Autodesk Inventor part; units mm, degrees
ref_plane "Work Plane1" through (10, 0, 0) normal (1, 0, 0) x (0, 0, -1)
ref_plane "YZ Plane" through (0, 0, 0) normal (1, 0, 0) x (0, 1, 0)
ref_plane "XZ Plane" through (0, 0, 0) normal (0, 1, 0) x (-1, 0, 0)
sketch "Sketch1" plane through (0, 0, 0) normal (0, 0, 1) x (1, 0, 0)
  line L0 (0, 0) -> (20, 0)
  line L1 (20, 0) -> (20, 31)
  line L2 (20, 31) -> (0, 31)
  line L3 (0, 31) -> (0, 0)
  dimension "d0" = 20
  dimension "d1" = 31
extrude "Extrusion1" add sketch "Sketch1" along normal blind 7
sketch "Sketch2" plane through (0, 0, 7) normal (0, 0, 1) x (1, 0, 0)
  line L0 (20, 31) -> (0, 31)
  line L1 (2, 31) -> (18, 31)
  line L2 (18, 31) -> (18, 11)
  line L3 (18, 11) -> (2, 11)
  line L4 (2, 11) -> (2, 31)
  line L5 (0, 31) -> (0, 0)
  line L6 (20, 0) -> (20, 31)
  dimension "d4" = 20
  dimension "d5" = 2
  dimension "d6" = 2
extrude "Extrusion2" cut sketch "Sketch2" against normal blind 4.5
sketch "Sketch3" plane through (0, 0, 7) normal (0, 0, 1) x (1, 0, 0)
  line L0 (18, 11) -> (2, 11)
  line L1 (1, 0) -> (19, 0)
  line L2 (19, 0) -> (19, 11)
  line L3 (19, 11) -> (1, 11)
  line L4 (1, 11) -> (1, 0)
  line L5 (0, 31) -> (0, 0)
  line L6 (20, 0) -> (20, 31)
  dimension "d9" = 1
  dimension "d10" = 1
extrude "Extrusion3" cut sketch "Sketch3" against normal blind 3
sketch "Sketch4" plane through (0, 0, 2.5) normal (0, 0, 1) x (1, 0, 0)
  circle A0 centre (6.19, 15) radius 1.5
  circle A1 centre (13.81, 15) radius 1.5
  line L0 (19, 0) -> (1, 0)
  line L1 (2, 31) -> (18, 31)
  line L2 (2, 11) -> (2, 31) construction
  line L3 (2, 31) -> (18, 31) construction
  line L4 (2, 11) -> (2, 31) construction
  line L5 (18, 11) -> (2, 11) construction
  line L6 (18, 31) -> (18, 11) construction
  line L7 (20, 31) -> (0, 31) construction
  line L8 (10, 31) -> (10, 11) construction
  line L9 (18, 11) -> (2, 11) construction
  line L10 (10, 31) -> (30, 31) construction
  point P0 (0, 0)
  point P1 (2, 21)
  dimension "d13" = 3
  dimension "d14" = 3
  dimension "d15" = 7.62
  dimension "d16" = 15
  dimension "d17" = 90
extrude "Extrusion4" cut sketch "Sketch4" against normal up to next
chamfer "Chamfer1" distance 0.5 angle 45 2 edges at (4.69, 15, 2.5) (12.31, 15, 2.5)
sketch "Sketch5" plane through (20, 0, 0) normal (1, 0, 0) x (0, 0, -1)
  line L0 (0, 0) -> (-7, 0) construction
  line L1 (-3.5, 0) -> (-3.5, 31) construction
  line L2 (-3.5, 0) -> (27.5, 0) construction
  line L3 (-3.5, 5) -> (-3.5, 10) construction
  line L4 (-2, 5) -> (-2, 10)
  line L5 (-5, 10) -> (-5, 5)
  arc A0 (-5, 5) -> (-2, 5) centre (-3.5, 5) ccw
  arc A1 (-2, 10) -> (-5, 10) centre (-3.5, 10) ccw
  line L6 (-3.5, 21) -> (-3.5, 26) construction
  line L7 (-2, 21) -> (-2, 26)
  line L8 (-5, 26) -> (-5, 21)
  arc A2 (-5, 21) -> (-2, 21) centre (-3.5, 21) ccw
  arc A3 (-2, 26) -> (-5, 26) centre (-3.5, 26) ccw
  line L9 (0, 31) -> (-7, 31)
  point P0 (-3.5, 7.5)
  point P1 (-3.5, 23.5)
  dimension "d23" = 31
  dimension "d24" = 90
  dimension "d25" = 3
  dimension "d26" = 3
  dimension "d27" = 5
  dimension "d28" = 5
  dimension "d29" = 5
  dimension "d30" = 5
extrude "Extrusion5" add sketch "Sketch5" along normal blind 1
ref_plane "Work Plane1" through (10, 0, 0) normal (1, 0, 0) x (0, 0, -1)
mirror "Mirror1" about plane through (10, 0, 0) normal (1, 0, 0) of "Extrusion5"
fillet "Fillet2" radius 1 16 edges at (21, 19.5, 3.5) (21, 23.5, 2) (21, 27.5, 3.5) (21, 23.5, 5) (21, 3.5, 3.5) (21, 7.5, 2) (21, 11.5, 3.5) (21, 7.5, 5) (-1, 19.5, 3.5) (-1, 23.5, 2) (-1, 27.5, 3.5) (-1, 23.5, 5) (-1, 3.5, 3.5) (-1, 7.5, 2) (-1, 11.5, 3.5) (-1, 7.5, 5)
fillet "Fillet3" radius 1 2 edges at (2, 21, 2.5) (18, 21, 2.5)
chamfer "Chamfer2" distance 0.5 angle 45 2 edges at (12.31, 15, 0) (4.69, 15, 0)
properties part number "Top"
CAD build for the part. Positions are in the model's coordinates, mm. A direction names the side the tool comes from. Give positions to 0.01 mm unless a question says otherwise; leave off trailing zeros. Loops run counter-clockwise (first coordinate to the right, second up) from the corner with the lowest first, then second, coordinate; pieces in that order, holes last. Notation, with made-up numbers: (30, -31) -> (65, -31) arc R11 cw to (65, -25) -> close; hole circle Ø7 at (34.5, 71.5). An arc over 180 degrees is marked (long way). Use a Markdown table: item, result.
1. Which spindle directions (+Z, -Z, +X, -X, +Y, -Y) get a long thin tool onto all of the face, cutting with end or side? Do faces 1 (the flat face through (18.5, 11, 5.5)), 2 (the flat face through (21, 23.5, 3.5)). Say none if no direction does.
Check result:
| item | result |
|---|---|
| face 1 | +Z, -Y |
| face 2 | +Z, -Z, +X, +Y, -Y |
2. Flat gauge pins, fed straight in: pin 1 (0.8 mm diameter, centred on x = 12, z = 3, fed in from +Y); pin 2 (0.8 mm diameter, centred on x = 1.5, z = 6, fed in from -Y); pin 3 (0.9 mm diameter, centred on y = 6, z = 6, fed in from +X); pin 4 (1.8 mm diameter, centred on x = 13.81, y = 15, fed in from +Z). Where does each tip first touch, or does it go through?
Check result:
| item | result |
|---|---|
| pin 1 | stops at y = 11 |
| pin 2 | stops at y = 11 |
| pin 3 | stops at x = 20 |
| pin 4 | passes through |
3. Slice it at B-B (y = 15). List the corners of the cut face in (x, z).
Check result:
| item | result |
|---|---|
| outline | (0, 0) -> (4.19, 0) -> (4.69, 0.5) -> (4.69, 2) -> (4.19, 2.5) -> (3, 2.5) arc R1 cw to (2, 3.5) -> (2, 7) -> (0, 7) -> close; (7.69, 0.5) -> (8.19, 0) -> (11.81, 0) -> (12.31, 0.5) -> (12.31, 2) -> (11.81, 2.5) -> (8.19, 2.5) -> (7.69, 2) -> close; (15.31, 0.5) -> (15.81, 0) -> (20, 0) -> (20, 7) -> (18, 7) -> (18, 3.5) arc R1 cw to (17, 2.5) -> (15.81, 2.5) -> (15.31, 2) -> close |
4. Wall check: L1, parallel to Y at x = 13.81, z = 1.6; L2, parallel to X at y = 18, z = 5.5; L3, parallel to X at y = 6, z = 5.5. Give the ranges that are in metal, low to high. Write a range as [from, to].
Check result:
| item | result |
|---|---|
| L1 | y = [0, 13.5], [16.5, 31] |
| L2 | x = [0, 2], [18, 20] |
| L3 | x = [0, 1], [19, 20] |
5. Mould opens along X. For faces 3 (the flat face through (1, 6, 6)), 4 (the flat face through (20, 15, 3)), 5 (the flat face through (10, 31, 2)) say: pulls with the +X half, pulls with the -X half, needs draft (parallel to the pull), parting line crosses it, or undercut.
Check result:
| item | result |
|---|---|
| face 3 | undercut |
| face 4 | pulls with the +X half |
| face 5 | needs draft |
6. Slice it at A-A (x = 6.19). List the corners of the cut face in (y, z).
Check result:
| item | result |
|---|---|
| outline | (0, 0) -> (13, 0) -> (13.5, 0.5) -> (13.5, 2) -> (13, 2.5) -> (11, 2.5) -> (11, 4) -> (0, 4) -> close; (16.5, 0.5) -> (17, 0) -> (31, 0) -> (31, 2.5) -> (17, 2.5) -> (16.5, 2) -> close |
7. Slice it at C-C (z = 6.5). List the corners of the cut face in (x, y), plus the area to 3 significant figures.
Check result:
| item | result |
|---|---|
| outline | (0, 0) -> (1, 0) -> (1, 11) -> (2, 11) -> (2, 31) -> (0, 31) -> close; (18, 11) -> (19, 11) -> (19, 0) -> (20, 0) -> (20, 31) -> (18, 31) -> close |
| area | 102 mm^2 |
